The listing builds one solid part. Answer for the finished solid, in the listing's coordinates (mm). Round coordinates to 2 decimals unless told otherwise and drop trailing zeros. Order: outer loops, then holes, each group sorted by start corner. A loop starts at its lowest first (then second) coordinate and runs counter-clockwise, first axis right, second up. Notation, with made-up numbers: M -28,62.5 L 21,62.5 A16 ccw 21,93.5 Z; hole C -23.5,-10.75 d10. An arc over 180 degrees is marked long. Write item = value, one per line. Start each with the question number.
(1) A cutting plane is placed at C-C, the plane y = -0.45. Determine the outline of the cut face in (x, z), and give its area (3 significant figures).
(2) This flat-tipped pin is pushed along its axis until it touches: pin 1 (1 mm diameter, centred on x = 17.5, z = 21.5, fed in from +Y). Where does it stop, or does it pass through?
(3) For a pull along Z with two mould halves and no side action, classify faces 1 (the face through (-58, -1, 29)), 2 (the face through (58, -1, -29)), 3 (the face through (1, 0, 0)) as released by +Z, released by -Z, zero draft, split by the parting line, or undercut.
(4) A cutting plane is placed at B-B, the plane z = 0. Count the separate pieces of the cut face and the enclosed holes in it, and give its area (3 significant figures).
(5) Straight lines are drawn through the part: probe 1 along X at (y, z) = (-1, 0); probe 2 along X at (y, z) = (-1, 8); probe 3 along Z at (x, y) = (35.5, -0.85). For each, find the intervals that lie inside material, in ascending order. Write a range as from..to.
from build123d import *

# Parameters (mm, degrees)
SKETCH1_R          = 10
BASE_FLANGE1_DEPTH = 2
FILLET1_R          = 1
FILLET2_R          = 1
FILLET3_R          = 1


# Sheet-metal steps are written as plain solids
with BuildPart() as part:
    # Sketch1 → Base-Flange1 (new body)
    with BuildSketch(Plane(origin=(0, 0, 0), x_dir=(1, 0, 0), z_dir=(0, 1, 0))):
        with BuildLine():
            Line((55, -30), (-55, -30))
            ThreePointArc((-55, -30), (-58.535533906, -28.535533906), (-60, -25))
            Line((-60, -25), (-60, 25))
            ThreePointArc((-60, 25), (-58.535533906, 28.535533906), (-55, 30))
            Line((-55, 30), (55, 30))
            ThreePointArc((55, 30), (58.535533906, 28.535533906), (60, 25))
            Line((60, 25), (60, -25))
            ThreePointArc((60, -25), (58.535533906, -28.535533906), (55, -30))
        make_face()
        with Locations(Location((-40, 0, 0), (0, 0, 270))):
            Circle(SKETCH1_R, mode=Mode.SUBTRACT)
        with Locations(Location((40, 0, 0), (0, 0, 270))):
            Circle(SKETCH1_R, mode=Mode.SUBTRACT)
    extrude(amount=-BASE_FLANGE1_DEPTH)

    # Fillet1
    fillet1_edges = [part.edges().sort_by_distance(p)[0] for p in [
        (-40, 0, -10),
        (40, 0, -10),
    ]]
    fillet(fillet1_edges, radius=FILLET1_R)

    # Fillet2
    fillet2_edges = [part.edges().sort_by_distance(p)[0] for p in [
        (-40, -2, -10),
    ]]
    fillet(fillet2_edges, radius=FILLET2_R - 0.0001)  # a hair under: the kernel refuses the full size

    # Fillet3
    fillet3_edges = [part.edges().sort_by_distance(p)[0] for p in [
        (40, -2, -10),
    ]]
    fillet(fillet3_edges, radius=FILLET3_R - 0.0001)  # a hair under: the kernel refuses the full size


solid = part.part
Reported:
q1.outline = M -60,-25 A5 ccw -55,-30 L 55,-30 A5 ccw 60,-25 L 60,25 A5 ccw 55,30 L -55,30 A5 ccw -60,25 Z; hole C -40,0 d20.33; hole C 40,0 d20.33
q1.area = 6,530 mm²
q2.pin_1 = 0
q3.face_1 = released by +Z
q3.face_2 = released by -Z
q3.face_3 = zero draft
q4.separate_pieces = 3
q4.enclosed_holes = 0
q4.area = 158 mm²
q5.probe_1 = -60..-50, -30..30, 50..60
q5.probe_2 = -60..-46, -34..34, 46..60
q5.probe_3 = -30..-8.94, 8.94..30
